```python
from build123d import *

# Parameters (mm, degrees)
BOSS_EXTRUDE1_DEPTH                 = 111.76
SKETCH5_W                           = 304.8
SKETCH5_H                           = 25.4
CUT_EXTRUDE3_DEPTH                  = 101.6
CUT_EXTRUDE4_DEPTH                  = 227.288199427
CUT_EXTRUDE4_DEPTH_BACK             = 227.288199427
SKETCH3_W                           = 96.52
SKETCH3_H                           = 101.6
SKETCH3_W_2                         = 48.26
CUT_EXTRUDE5_REACH                  = 288.663
SKETCH6_W                           = 38.1
SKETCH6_H                           = 50.8
SKETCH7_W                           = 81.28
SKETCH7_H                           = 50.8
BOSS_EXTRUDE2_DEPTH                 = 5.08
CUT_EXTRUDE6_REACH                  = 200.969
SKETCH8_R                           = 10.16
SKETCH9_W                           = 5.08
SKETCH9_H                           = 95.25
BOSS_EXTRUDE3_DEPTH                 = 10.16
SKETCH10_W                          = 5.08
SKETCH10_H                          = 95.206439839
BOSS_EXTRUDE4_DEPTH                 = 10.16
CUT_EXTRUDE7_REACH                  = 208.854
FILLET1_R                           = 50.8
BOSS_EXTRUDE5_REACH                 = 208.854
CUT_EXTRUDE8_REACH                  = 248.593
CUT_EXTRUDE8_END_RADIUS             = 126.32098656
CUT_EXTRUDE8_DIRECTION_2_REACH      = 248.593
CUT_EXTRUDE8_DIRECTION_2_END_RADIUS = 126.32098656


with BuildPart() as part:
    # Sketch1 → Boss-Extrude1 (new body)
    with BuildSketch(Plane.XY):
        Polygon((-152.4, 62.23), (-152.4, -33.02), (0, -62.23), (152.4, -32.976439839), (152.4, 62.23), align=None)
    extrude(amount=-BOSS_EXTRUDE1_DEPTH)

    # Sketch5 → Cut-Extrude3 (cut)
    with BuildSketch(Plane.XY.offset(-5.08)):
        with Locations((0, -1.27)):
            Rectangle(SKETCH5_W, SKETCH5_H)
    extrude(amount=-CUT_EXTRUDE3_DEPTH, mode=Mode.SUBTRACT)

    # Sketch3 → Cut-Extrude4 (cut, two sides: drawn at the far end of the back side and taken through both)
    with BuildSketch(Plane(origin=(0, 62.23, 0), x_dir=(1, 0, 0), z_dir=(0, 1, 0)).offset(-CUT_EXTRUDE4_DEPTH_BACK)):
        with Locations((-50.8, 55.88)):
            Rectangle(SKETCH3_W, SKETCH3_H)
        with Locations((50.8, 55.88)):
            Rectangle(SKETCH3_W, SKETCH3_H)
        with Locations((-128.27, 55.88)):
            Rectangle(SKETCH3_W_2, SKETCH3_H)
        with Locations((128.27, 55.88)):
            Rectangle(SKETCH3_W_2, SKETCH3_H)
    extrude(amount=CUT_EXTRUDE4_DEPTH + CUT_EXTRUDE4_DEPTH_BACK, mode=Mode.SUBTRACT)

    # Cut-Extrude5: up to this face of the body (flat: up to its plane)
    cut_extrude5_end = Plane(part.part.faces().sort_by_distance((104.14, 36.83, -55.88))[0])
    # Sketch6 → Cut-Extrude5 (cut, up to the picked face)
    with BuildSketch(Plane.ZY.offset(104.14), mode=Mode.PRIVATE) as cut_extrude5_sk1:
        with Locations((-55.932057734, 36.83)):
            Rectangle(SKETCH6_W, SKETCH6_H)
    cut_extrude5_tool1 = split(extrude(cut_extrude5_sk1.sketch, amount=-CUT_EXTRUDE5_REACH, mode=Mode.PRIVATE), bisect_by=cut_extrude5_end, keep=Keep.BOTH, mode=Mode.PRIVATE)
    add(cut_extrude5_tool1.solids().sort_by(Axis((-104.14, 36.83, -55.932058), (1, 0, 0)))[0], mode=Mode.SUBTRACT)

    # Sketch7 → Boss-Extrude2 (add)
    with BuildSketch(Plane(origin=(0, 0, -36.882057734), x_dir=(-1, 0, 0), z_dir=(0, 0, -1))):
        with Locations((0, 36.83)):
            Rectangle(SKETCH7_W, SKETCH7_H)
        with Locations((101.6, 36.83)):
            Rectangle(SKETCH7_W, SKETCH7_H)
        with Locations((-101.6, 36.83)):
            Rectangle(SKETCH7_W, SKETCH7_H)
    boss_extrude2 = extrude(amount=-BOSS_EXTRUDE2_DEPTH)

    # Mirror1: Boss-Extrude2 across plane
    add(boss_extrude2.mirror(Plane(origin=(0, 0, -55.932057734), x_dir=(1, 0, 0), z_dir=(0, 0, -1))))

    # Cut-Extrude6: up to this face of the body (flat: up to its plane)
    cut_extrude6_end = Plane(part.part.faces().sort_by_distance((-0.010072712, 6.983811852, -111.76))[0])
    # Sketch8 → Cut-Extrude6 (cut, up to the picked face)
    with BuildSketch(Plane.XY, mode=Mode.PRIVATE) as cut_extrude6_sk1:
        with Locations((50.8, 36.83)):
            Circle(SKETCH8_R)
    cut_extrude6_tool1 = split(extrude(cut_extrude6_sk1.sketch, amount=-CUT_EXTRUDE6_REACH, mode=Mode.PRIVATE), bisect_by=cut_extrude6_end, keep=Keep.BOTH, mode=Mode.PRIVATE)
    cut_extrude6 = cut_extrude6_tool1.solids().sort_by(Axis((50.8, 36.83, 0), (0, 0, -1)))[0]
    add(cut_extrude6, mode=Mode.SUBTRACT)

    # Mirror2: Cut-Extrude6 across plane
    add(cut_extrude6.mirror(Plane(origin=(0, 0, 0), x_dir=(0, 0, 1), z_dir=(1, 0, 0))), mode=Mode.SUBTRACT)

    # Sketch9 → Boss-Extrude3 (add)
    with BuildSketch(Plane.ZY.offset(152.4)):
        with Locations((-109.22, 14.605)):
            Rectangle(SKETCH9_W, SKETCH9_H)
        with Locations((-2.54, 14.605)):
            Rectangle(SKETCH9_W, SKETCH9_H)
    extrude(amount=BOSS_EXTRUDE3_DEPTH)

    # Sketch10 → Boss-Extrude4 (add)
    with BuildSketch(Plane(origin=(152.4, 0, 0), x_dir=(0, 0, -1), z_dir=(1, 0, 0))):
        with Locations((2.54, 14.626780081)):
            Rectangle(SKETCH10_W, SKETCH10_H)
        with Locations((109.22, 14.626780081)):
            Rectangle(SKETCH10_W, SKETCH10_H)
    extrude(amount=BOSS_EXTRUDE4_DEPTH)

    # Cut-Extrude7: up to this face of the body (flat: up to its plane)
    cut_extrude7_end = Plane(part.part.faces().sort_by_distance((-0.011704667, 6.851805545, -111.76))[0])
    # Sketch11 → Cut-Extrude7 (cut, up to the picked face)
    with BuildSketch(Plane.XY, mode=Mode.PRIVATE) as cut_extrude7_sk1:
        Polygon((-162.56, -12.7), (-119.696308585, -39.288207521), (-152.4, -33.02), (-162.56, -33.02), align=None)
    cut_extrude7_tool1 = split(extrude(cut_extrude7_sk1.sketch, amount=-CUT_EXTRUDE7_REACH, mode=Mode.PRIVATE), bisect_by=cut_extrude7_end, keep=Keep.BOTH, mode=Mode.PRIVATE)
    # Sketch11 → Cut-Extrude7 (cut, up to the picked face)
    with BuildSketch(Plane.XY, mode=Mode.PRIVATE) as cut_extrude7_sk2:
        Polygon((152.4, -33.02), (162.56, -33.02), (162.56, -12.7), (119.696308585, -39.288207521), align=None)
    cut_extrude7_tool2 = split(extrude(cut_extrude7_sk2.sketch, amount=-CUT_EXTRUDE7_REACH, mode=Mode.PRIVATE), bisect_by=cut_extrude7_end, keep=Keep.BOTH, mode=Mode.PRIVATE)
    add(cut_extrude7_tool1.solids().sort_by(Axis((-148.539263, -27.801749, 0), (0, 0, -1)))[0], mode=Mode.SUBTRACT)
    add(cut_extrude7_tool2.solids().sort_by(Axis((148.539263, -27.801749, 0), (0, 0, -1)))[0], mode=Mode.SUBTRACT)

    # Fillet1
    # the kernel refuses this fillet: 50.8 mm, written as the material it takes off along each edge
    with BuildSketch(Plane(origin=(-162.56, -12.7, 70.671047804), x_dir=(0.8497897447130388, -0.5271217978613181, 0), z_dir=(0, 0, -1)), Plane(origin=(-162.56, -12.7, -36.008952196), x_dir=(0.8497897447130388, -0.5271217978613181, 0), z_dir=(0, 0, -1)), Plane(origin=(162.56, -12.7, 70.671047804), x_dir=(0, 1, 0), z_dir=(0, 0, -1))) as fillet1_piece_1:
        with BuildLine():
            CenterArc((FILLET1_R * 0.556464943335, -FILLET1_R), FILLET1_R, 90, 58.188808221)
            Line((-FILLET1_R * 0.293324801378, -FILLET1_R * 0.472878202139), (0, 0))
            Line((0, 0), (FILLET1_R * 0.556464943335, 0))
        make_face()
    extrude(amount=146.422095607, mode=Mode.SUBTRACT)
    with BuildSketch(Plane(origin=(-119.696308585, -39.288207521, -83.186546401), x_dir=(0.9821230119270369, -0.18824024395268216, 0), z_dir=(0, 0, -1)), Plane(origin=(-119.696308585, -39.288207521, 23.493453599), x_dir=(0.9821230119270369, -0.18824024395268216, 0), z_dir=(0, 0, -1))) as fillet1_piece_2:
        with BuildLine():
            CenterArc((FILLET1_R * 0.184987823618, -FILLET1_R), FILLET1_R, 90, 20.961087149)
            Line((-FILLET1_R * 0.172745995297, -FILLET1_R * 0.0661764005955), (0, 0))
            Line((0, 0), (FILLET1_R * 0.184987823618, 0))
        make_face()
    extrude(amount=52.066907199, mode=Mode.SUBTRACT)
    with BuildSketch(Plane(origin=(162.56, -12.7, -36.008952196), x_dir=(-0.8497897447130388, -0.5271217978613181, 0), z_dir=(0, 0, -1))) as fillet1_piece_3:
        with BuildLine():
            CenterArc((FILLET1_R * 0.556464943335, FILLET1_R), FILLET1_R, 211.811191779, 58.188808221)
            Line((-FILLET1_R * 0.293324801378, FILLET1_R * 0.472878202139), (0, 0))
            Line((0, 0), (FILLET1_R * 0.556464943335, 0))
        make_face()
    extrude(amount=146.422095607, mode=Mode.SUBTRACT)
    with BuildSketch(Plane(origin=(119.776180176, -39.238663434, 23.475348992), x_dir=(-0.9820710795721669, -0.18851099349363817, 0), z_dir=(0, 0, -1)), Plane(origin=(119.776180176, -39.238663434, -83.204651008), x_dir=(-0.9820710795721669, -0.18851099349363817, 0), z_dir=(0, 0, -1))) as fillet1_piece_4:
        with BuildLine():
            CenterArc((FILLET1_R * 0.184845267653, FILLET1_R), FILLET1_R, 249.054708445, 20.945291555)
            Line((-FILLET1_R * 0.172631096402, FILLET1_R * 0.0660778141933), (0, 0))
            Line((0, 0), (FILLET1_R * 0.184845267653, 0))
        make_face()
    extrude(amount=52.030697984, mode=Mode.SUBTRACT)
    with BuildSketch(Plane(origin=(0, -62.23, 24.359816254), x_dir=(-0.982123011927037, 0.1882402439526816, 0), z_dir=(0, 0, -1))) as fillet1_piece_5:
        with BuildLine():
            CenterArc((FILLET1_R * 0.191809576801, FILLET1_R), FILLET1_R, 248.283995147, 21.716004853)
            Line((-FILLET1_R * 0.178196707507, FILLET1_R * 0.0709707488072), (0, 0))
            Line((0, 0), (FILLET1_R * 0.191809576801, 0))
        make_face()
    extrude(amount=160.479632508, mode=Mode.SUBTRACT)

    # Boss-Extrude5: up to this face of the body (flat: up to its plane)
    boss_extrude5_end = Plane(part.part.faces().sort_by_distance((-0.004823682, 7.831331811, -111.76))[0])
    # Sketch12 → Boss-Extrude5 (add, up to the picked face)
    with BuildSketch(Plane.XY, mode=Mode.PRIVATE) as boss_extrude5_sk1:
        with BuildLine():
            Line((-162.56, 62.23), (-210.82, 62.23))
            ThreePointArc((-210.82, 62.23), (-185.525923559, 8.586514121), (-138.537787331, -27.60089991))
            Line((-138.537787331, -27.60089991), (-162.56, 62.23))
        make_face()
    boss_extrude5_tool1 = split(extrude(boss_extrude5_sk1.sketch, amount=-BOSS_EXTRUDE5_REACH, mode=Mode.PRIVATE), bisect_by=boss_extrude5_end, keep=Keep.BOTH, mode=Mode.PRIVATE)
    # Sketch12 → Boss-Extrude5 (add, up to the picked face)
    with BuildSketch(Plane.XY, mode=Mode.PRIVATE) as boss_extrude5_sk2:
        with BuildLine():
            Line((162.56, 62.23), (210.82, 62.23))
            ThreePointArc((210.82, 62.23), (185.525923559, 8.586514121), (138.537787331, -27.60089991))
            Line((138.537787331, -27.60089991), (162.56, 62.23))
        make_face()
    boss_extrude5_tool2 = split(extrude(boss_extrude5_sk2.sketch, amount=-BOSS_EXTRUDE5_REACH, mode=Mode.PRIVATE), bisect_by=boss_extrude5_end, keep=Keep.BOTH, mode=Mode.PRIVATE)
    add(boss_extrude5_tool1.solids().sort_by(Axis((-173.436994, 26.131053, 0), (0, 0, -1)))[0])
    add(boss_extrude5_tool2.solids().sort_by(Axis((173.436994, 26.131053, 0), (0, 0, -1)))[0])

    # Cut-Extrude8: up to this cylinder (the profile starts inside it)
    cut_extrude8_end = Plane(origin=(-87.109319049, 87.777192878, -55.90231), z_dir=(0, 0, 1)) * Cylinder(CUT_EXTRUDE8_END_RADIUS, 750.827973119, mode=Mode.PRIVATE)
    # Sketch13 → Cut-Extrude8 (cut, up to the surface)
    with BuildSketch(Plane(origin=(0, 0, 0), x_dir=(0, 0, -1), z_dir=(1, 0, 0)), mode=Mode.PRIVATE) as cut_extrude8_sk1:
        Polygon((36.882057734, 62.23), (36.882057734, 11.43), (5.08, 11.43), (5.08, -13.97), (106.68, -13.97), (106.68, 11.43), (74.982057734, 11.43), (74.982057734, 62.23), align=None)
    cut_extrude8_tool1 = extrude(cut_extrude8_sk1.sketch, amount=-CUT_EXTRUDE8_REACH, mode=Mode.PRIVATE) & cut_extrude8_end
    add(cut_extrude8_tool1.solids().sort_by_distance((0, 15.058571, -55.90231))[0], mode=Mode.SUBTRACT)

    # Cut-Extrude8 direction 2: up to this cylinder (the profile starts inside it)
    cut_extrude8_direction_2_end = Plane(origin=(87.109319049, 87.777192878, -55.90231), z_dir=(0, 0, 1)) * Cylinder(CUT_EXTRUDE8_DIRECTION_2_END_RADIUS, 750.827973119, mode=Mode.PRIVATE)
    # Sketch13 → Cut-Extrude8 direction 2 (cut, up to the surface)
    with BuildSketch(Plane(origin=(0, 0, 0), x_dir=(0, 0, -1), z_dir=(1, 0, 0)), mode=Mode.PRIVATE) as cut_extrude8_direction_2_sk1:
        Polygon((36.882057734, 62.23), (36.882057734, 11.43), (5.08, 11.43), (5.08, -13.97), (106.68, -13.97), (106.68, 11.43), (74.982057734, 11.43), (74.982057734, 62.23), align=None)
    cut_extrude8_direction_2_tool1 = extrude(cut_extrude8_direction_2_sk1.sketch, amount=CUT_EXTRUDE8_DIRECTION_2_REACH, mode=Mode.PRIVATE) & cut_extrude8_direction_2_end
    add(cut_extrude8_direction_2_tool1.solids().sort_by_distance((0, 15.058571, -55.90231))[0], mode=Mode.SUBTRACT)


solid = part.part
```
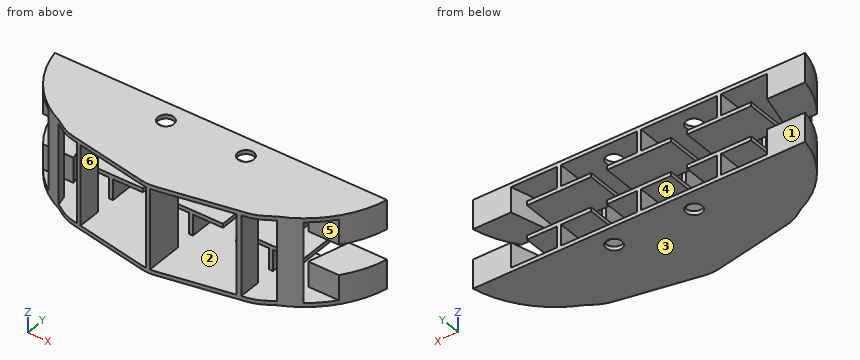
The listing builds one solid part. Answer for the finished solid, in the listing's coordinates (mm). Face numbers are marked on the shaded views. A direction names the side the tool comes from. Coordinates: 2 decimals unless noted, no trailing zeros. Order: outer loops, then holes, each group sorted by start corner. A loop starts at its lowest first (then second) coordinate and runs counter-clockwise, first axis right, second up. Notation, with made-up numbers: M -13,-34.75 L 19,-34.75 A8 ccw 19,-26.75 Z; hole C 75.5,-28.5 d1. An arc over 180 degrees is marked long. Answer as a JSON object with one key per item and string values. Group by question number.
1. Flat-ended cylindrical pins translate along their axes: P1, Ø2, axis at y = -29, z = -73.5, coming from the +X side; P2, Ø14, axis at y = -32.5, z = -49.5, coming from the +X side; P3, Ø4, axis at y = 37, z = -77.5, coming from the +X side; P4, Ø16, axis at x = 149, z = -80.5, coming from the +Y side. Find the tip coordinate at first contact, or state that the pin passes through.
2. Section C-C on z = -20.5 is taken. State how many separate pieces and enclosed holes the cut face has, then the cut area to 3 significant figures.
3. A tool of negligible diameter and unlimited length cuts with its end or side. For the marked faces 4, 5 and 6, from which of +Z, -Z, +X, -X, +Y, -Y can it reach the whole face along a straight path? Write none if from no direction.
4. Determine the mould class of the marked faces 1, 2 and 3 for opening direction Z: released by +Z, released by -Z, zero draft, split by the parting line, or undercut.
5. Section B-B on x = 50.8 is taken. Write down the section's boundary in (y, z), then the cut area to 3 significant figures.
6. Section A-A on y = -1.5 is taken. Write down the section's boundary in (x, z).
7. Straight lines are drawn through the part: line 1 (Z direction, x = 71, y = 23); line 2 (X direction, y = -38.5, z = -79.5); line 3 (Z direction, x = -1, y = 6). For each, find the intervals that lie inside material, in ascending order.
8. Section D-D on y = -50 is taken. Write down the section's boundary in (x, z), then the cut area to 3 significant figures.
Values follow:
{
 "1": {"P1": "x = 104.14", "P2": "x = 143.01", "P3": "x = 203.63", "P4": "y = 62.23"},
 "2": {"separate pieces": "10", "enclosed holes": "0", "area": "6,260 mm2"},
 "3": {"face 4": "+Y, -Y", "face 5": "+X, -X", "face 6": "-Y"},
 "4": {"face 1": "zero draft", "face 2": "undercut", "face 3": "released by -Z"},
 "5": {"outline": "M -52.48,-111.76 L 26.67,-111.76 L 26.67,-106.68 L -52.48,-106.68 Z; M -52.48,-5.08 L 26.67,-5.08 L 26.67,0 L -52.48,0 Z; M 46.99,-111.76 L 62.23,-111.76 L 62.23,-106.68 L 46.99,-106.68 Z; M 46.99,-5.08 L 62.23,-5.08 L 62.23,0 L 46.99,0 Z", "area": "959 mm2"},
 "6": {"outline": "M -176.48,-111.76 L 176.48,-111.76 L 176.48,-106.68 L -176.48,-106.68 Z; M -176.48,-5.08 L 176.48,-5.08 L 176.48,0 L -176.48,0 Z"},
 "7": {"line 1": "-111.76 to -106.68, -80.06 to -74.98, -36.88 to -31.8, -5.08 to 0", "line 2": "-104.14 to -99.06, -2.54 to 2.54, 99.06 to 104.14", "line 3": "-111.76 to -106.68, -5.08 to 0"},
 "8": {"outline": "M -63.81,-111.76 L 63.71,-111.76 L 63.71,-106.68 L 2.54,-106.68 L 2.54,-5.08 L 63.71,-5.08 L 63.71,0 L -63.81,0 L -63.81,-5.08 L -2.54,-5.08 L -2.54,-106.68 L -63.81,-106.68 Z", "area": "1,810 mm2"}
}
